Model file for the job. Use its own axes, mm. A direction names the side the tool comes from. Coordinates: 2 decimals unless noted, no trailing zeros. Write each loop counter-clockwise with the first axis right and the second up, starting at its lowest first coordinate (ties: lowest second). Pieces come first, ordered by that corner, then holes.
Q1. Pull direction X, two halves, no side cores. Call faces 4 (the flat face through (46.505, 4, 1)), 5 (the cylindrical face through (22.5, 3.5, 1.5)), 6 (the flat face through (-13, 0, 1)): released by +X, released by -X, zero draft, split by the parting line, or undercut.
Q2. Which spindle directions (+Z, -Z, +X, -X, +Y, -Y) get a long thin tool onto all of the face, cutting with end or side? Do faces 1 (the cylindrical face through (-18.84, 6.52, 1.48)), 2 (the flat face through (35, 0, 1)), 3 (the flat face through (-15.995, 5, 1)). Say none if no direction does.
Q3. Drill centre lines: probe 1 along X at (y, z) = (-0.5, 1); probe 2 along X at (y, z) = (4.75, 0.3) (3 decimals); probe 3 along Y at (x, z) = (0, 2.85). Where is each one in solid material? Low to high.
Q4. Band-saw the part on C-C, the plane z = 2.3. Write the cut outline in (x, y) (3 decimals), plus the area to 3 significant figures.
Q5. Band-saw the part on B-B, the plane x = 22.51. Write the cut outline in (y, z), plus the area to 3 significant figures.
Q6. Band-saw the part on D-D, the plane x = 2.5. Write the cut outline in (y, z), plus the area to 3 significant figures.
Q7. Pin check, flat tips, straight feed: P1, Ø5, axis at x = 0, y = 0, coming from the -Z side; P2, Ø2, axis at x = 42.505, y = 7, coming from the +Z side; P3, Ø1, axis at x = 9, z = 1, coming from the +Y side; P4, Ø0.9, axis at x = 37, z = 1, coming from the -Y side. Stop position of each tip, or through.
Q8. Band-saw the part on A-A, the plane y = 4.75. Write the cut outline in (x, z) (3 decimals), plus the area to 3 significant figures.
from build123d import *

# Parameters (mm, degrees)
SKETCH_1_R      = 1.5
SKETCH_1_R_2    = 1.25
EXTRUDE_2_DEPTH = 3


with BuildPart() as part:
    # 草图1 → 凸台-拉伸2 (new body)
    with BuildSketch(Plane.XY):
        with BuildLine():
            Line((3.5, 0), (19.01, 0))
            ThreePointArc((19.01, 0), (22.51, -3.5), (26.01, 0))
            Line((26.01, 0), (44.505, 0))
            Line((44.505, 0), (46.505, 2))
            Line((46.505, 2), (46.505, 7))
            ThreePointArc((46.505, 7), (42.505, 11), (38.505, 7))
            Line((38.505, 7), (38.505, 3))
            Line((38.505, 3), (24.312775638, 3))
            ThreePointArc((24.312775638, 3), (22.51, 3.5), (20.707224362, 3))
            Line((20.707224362, 3), (1.802775638, 3))
            ThreePointArc((1.802775638, 3), (0, 3.5), (-1.802775638, 3))
            Line((-1.802775638, 3), (-15.995, 3))
            Line((-15.995, 3), (-15.995, 7))
            ThreePointArc((-15.995, 7), (-19.995, 11), (-23.995, 7))
            Line((-23.995, 7), (-23.995, 2))
            Line((-23.995, 2), (-21.995, 0))
            Line((-21.995, 0), (-3.5, 0))
            ThreePointArc((-3.5, 0), (0, -3.5), (3.5, 0))
        make_face()
        with Locations((22.51, 0)):
            Circle(SKETCH_1_R, mode=Mode.SUBTRACT)
        Circle(SKETCH_1_R, mode=Mode.SUBTRACT)
        with Locations((-19.995, 7)):
            Circle(SKETCH_1_R_2, mode=Mode.SUBTRACT)
        with Locations((42.505, 7)):
            Circle(SKETCH_1_R_2, mode=Mode.SUBTRACT)
    extrude(amount=EXTRUDE_2_DEPTH)


solid = part.part
Answer sheet:
1. face 4: released by +X
1. face 5: undercut
1. face 6: zero draft
2. face 1: +Z, -Z
2. face 2: +Z, -Z, +X, -Y
2. face 3: +Z, -Z, +Y
3. probe 1: x = -3.46 to -1.41, 1.41 to 3.46, 19.05 to 21.1, 23.92 to 25.97
3. probe 2: x = -23.995 to -15.995, 38.505 to 46.505
3. probe 3: y = -3.5 to -1.5, 1.5 to 3.5
4. outline: (-23.995, 2) - (-21.995, 0) - (-3.5, 0) arc R3.5 ccw to (3.5, 0) - (19.01, 0) arc R3.5 ccw to (26.01, 0) - (44.505, 0) - (46.505, 2) - (46.505, 7) arc R4 ccw to (38.505, 7) - (38.505, 3) - (24.313, 3) arc R3.5 ccw to (20.707, 3) - (1.803, 3) arc R3.5 ccw to (-1.803, 3) - (-15.995, 3) - (-15.995, 7) arc R4 ccw to (-23.995, 7) - close; hole circle Ø2.5 at (-19.995, 7); hole circle Ø3 at (0, 0); hole circle Ø3 at (22.51, 0); hole circle Ø2.5 at (42.505, 7)
4. area: 339 mm2
5. outline: (-3.5, 0) - (-1.5, 0) - (-1.5, 3) - (-3.5, 3) - close; (1.5, 0) - (3.5, 0) - (3.5, 3) - (1.5, 3) - close
5. area: 12.0 mm2
6. outline: (-2.45, 0) - (3, 0) - (3, 3) - (-2.45, 3) - close
6. area: 16.3 mm2
7. P1: stops at z = 0
7. P2: passes through
7. P3: stops at y = 3
7. P4: stops at y = 0
8. outline: (-23.995, 0) - (-15.995, 0) - (-15.995, 3) - (-23.995, 3) - close; (38.505, 0) - (46.505, 0) - (46.505, 3) - (38.505, 3) - close
8. area: 48.0 mm2
